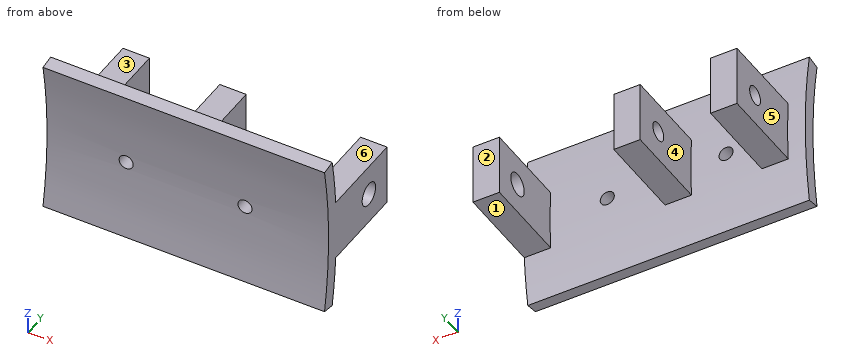
```python
from build123d import *

# Parameters (mm, degrees)
BASE_SKETCH_W           = 64
BASE_SKETCH_H           = 3
BASE_ANGLE              = 20
UPPER_EAR_SKETCH_W      = 6
UPPER_EAR_SKETCH_H      = 20.8
UPPER_EAR_DEPTH         = 7
LOWER_EAR_SKETCH_W      = 6
LOWER_EAR_SKETCH_H      = 20.8
LOWER_EAR_DEPTH         = 7
STOP_SKETCH_W           = 6
STOP_SKETCH_H           = 20.8
STOP_DEPTH              = 7
UPPER_EAR_HOLE_SKETCH_R = 2.1
UPPER_EAR_HOLE_DEPTH    = 6
LOWER_EAR_HOLE_SKETCH_R = 2.1
LOWER_EAR_HOLE_DEPTH    = 6
STOP_HOLE_SKETCH_R      = 2.6
STOP_HOLE_DEPTH         = 6
SCREW_HOLE_0_SKETCH_R   = 1.6
SCREW_HOLE_0_DEPTH      = 200
SCREW_HOLE_1_SKETCH_R   = 1.6
SCREW_HOLE_1_DEPTH      = 200


with BuildPart() as part:
    # Base Sketch → Base (revolve, symmetric)
    with BuildSketch(Plane.XY) as base_sk:
        with Locations((-598, 103.2)):
            Rectangle(BASE_SKETCH_W, BASE_SKETCH_H)
    revolve(axis=Axis((-3000, 0, 0), (1, 0, 0)), revolution_arc=BASE_ANGLE / 2)
    revolve(base_sk.sketch, axis=Axis((-3000, 0, 0), (-1, 0, 0)), revolution_arc=BASE_ANGLE / 2)

    # Upper Ear Sketch → Upper Ear (add, symmetric)
    with BuildSketch(Plane.XY):
        with Locations((-623, 113.9)):
            Rectangle(UPPER_EAR_SKETCH_W, UPPER_EAR_SKETCH_H)
    extrude(amount=UPPER_EAR_DEPTH, both=True)

    # Lower Ear Sketch → Lower Ear (add, symmetric)
    with BuildSketch(Plane.XY):
        with Locations((-601, 113.9)):
            Rectangle(LOWER_EAR_SKETCH_W, LOWER_EAR_SKETCH_H)
    extrude(amount=LOWER_EAR_DEPTH, both=True)

    # Stop Sketch → Stop (add, symmetric)
    with BuildSketch(Plane.XY):
        with Locations((-569, 113.9)):
            Rectangle(STOP_SKETCH_W, STOP_SKETCH_H)
    extrude(amount=STOP_DEPTH, both=True)

    # Upper Ear Hole Sketch → Upper Ear Hole (cut)
    with BuildSketch(Plane(origin=(-626, 0, 0), x_dir=(0, 0, -1), z_dir=(1, 0, 0))):
        with Locations((0, 117.3)):
            Circle(UPPER_EAR_HOLE_SKETCH_R)
    extrude(amount=UPPER_EAR_HOLE_DEPTH, mode=Mode.SUBTRACT)

    # Lower Ear Hole Sketch → Lower Ear Hole (cut)
    with BuildSketch(Plane(origin=(-604, 0, 0), x_dir=(0, 0, -1), z_dir=(1, 0, 0))):
        with Locations((0, 117.3)):
            Circle(LOWER_EAR_HOLE_SKETCH_R)
    extrude(amount=LOWER_EAR_HOLE_DEPTH, mode=Mode.SUBTRACT)

    # Stop Hole Sketch → Stop Hole (cut)
    with BuildSketch(Plane(origin=(-572, 0, 0), x_dir=(0, 0, -1), z_dir=(1, 0, 0))):
        with Locations((0, 117.3)):
            Circle(STOP_HOLE_SKETCH_R)
    extrude(amount=STOP_HOLE_DEPTH, mode=Mode.SUBTRACT)

    # Screw Hole 0 Sketch → Screw Hole 0 (cut)
    with BuildSketch(Plane(origin=(0, 0, 0), x_dir=(-1, 0, 0), z_dir=(0, 1, 0))):
        with Locations(Location((585, 0, 0), (0, 0, 270))):
            Circle(SCREW_HOLE_0_SKETCH_R)
    extrude(amount=SCREW_HOLE_0_DEPTH, mode=Mode.SUBTRACT)

    # Screw Hole 1 Sketch → Screw Hole 1 (cut)
    with BuildSketch(Plane(origin=(0, 0, 0), x_dir=(-1, 0, 0), z_dir=(0, 1, 0))):
        with Locations(Location((612, 0, 0), (0, 0, 270))):
            Circle(SCREW_HOLE_1_SKETCH_R)
    extrude(amount=SCREW_HOLE_1_DEPTH, mode=Mode.SUBTRACT)


solid = part.part
```
Verification items for the finished model (mm, model axes). Face numbers are marked on the shaded views. A direction names the side the tool comes from. Round coordinates to 2 decimals unless told otherwise and drop trailing zeros. Write each loop counter-clockwise with the first axis right and the second up, starting at its lowest first coordinate (ties: lowest second). Pieces come first, ordered by that corner, then holes.
1. Scan lines: L1, parallel to X at y = 116.75, z = 6; L2, parallel to X at y = 103.3, z = 0; L3, parallel to Y at x = -623.9, z = 0. Record each from-to range of solid material in increasing order.
2. Section check C-C on x = -623. Enter the section's corners in (y, z), plus the area to 3 significant figures.
3. Section check A-A on z = 0. State how many separate pieces and enclosed holes the cut face has, plus the area to 3 significant figures.
4. Section check B-B on y = 117.3. Enter the section's corners in (x, z), plus the area to 3 significant figures.
5. Draft check along X on the marked faces 4, 5 and 6. Enter one of: +X half, -X half, draft (parallel to the pull), parting line (faces both ways), or undercut.
6. Access from +Z, -Z, +X, -X, +Y, -Y to the whole of each face (thin tool, end or side, straight path). Record for the marked faces 1, 2 and 3.
7. Section check D-D on x = -585. Enter the section's corners in (y, z), plus the area to 3 significant figures.
8. Gauge pin test, flat ends, axial feed: P1, Ø2, axis at x = -596.5, z = -9, coming from the +Y side; P2, Ø1.8, axis at x = -624, y = 112.5, coming from the +Z side; P3, Ø2.5, axis at x = -612, z = 0, coming from the +Y side; P4, Ø4, axis at y = 110.5, z = -1.5, coming from the -X side. Record the tip position at first contact, or that the pin passes through.
Answer:
1. L1: x = -626 to -620, -604 to -598, -572 to -566
1. L2: x = -630 to -613.6, -610.4 to -586.6, -583.4 to -566
1. L3: y = 101.7 to 115.2, 119.4 to 124.3
2. outline: (100.15, -17.66) - (103.11, -18.18) arc R104.7 ccw to (104.47, -7) - (124.3, -7) - (124.3, 7) - (104.47, 7) arc R104.7 ccw to (103.11, 18.18) - (100.15, 17.66) arc R101.7 cw to start; hole circle Ø4.2 at (117.3, 0)
2. area: 370 mm2
3. separate pieces: 6
3. enclosed holes: 0
3. area: 444 mm2
4. outline: (-626, -7) - (-620, -7) - (-620, -2.1) - (-626, -2.1) - close; (-626, 2.1) - (-620, 2.1) - (-620, 7) - (-626, 7) - close; (-604, -7) - (-598, -7) - (-598, -2.1) - (-604, -2.1) - close; (-604, 2.1) - (-598, 2.1) - (-598, 7) - (-604, 7) - close; (-572, -7) - (-566, -7) - (-566, -2.6) - (-572, -2.6) - close; (-572, 2.6) - (-566, 2.6) - (-566, 7) - (-572, 7) - close
4. area: 170 mm2
5. face 4: undercut
5. face 5: -X half
5. face 6: draft
6. face 1: -Z, +X, -X, +Y
6. face 2: +Z, -Z, +X, -X, +Y
6. face 3: +Z, +X, -X, +Y
7. outline: (100.15, -17.66) - (103.11, -18.18) arc R104.7 ccw to (104.69, -1.6) - (101.69, -1.6) arc R101.7 cw to start; (100.15, 17.66) arc R101.7 cw to (101.69, 1.6) - (104.69, 1.6) arc R104.7 ccw to (103.11, 18.18) - close
7. area: 98.5 mm2
8. P1: stops at y = 104.39
8. P2: stops at z = 7
8. P3: passes through
8. P4: stops at x = -626
